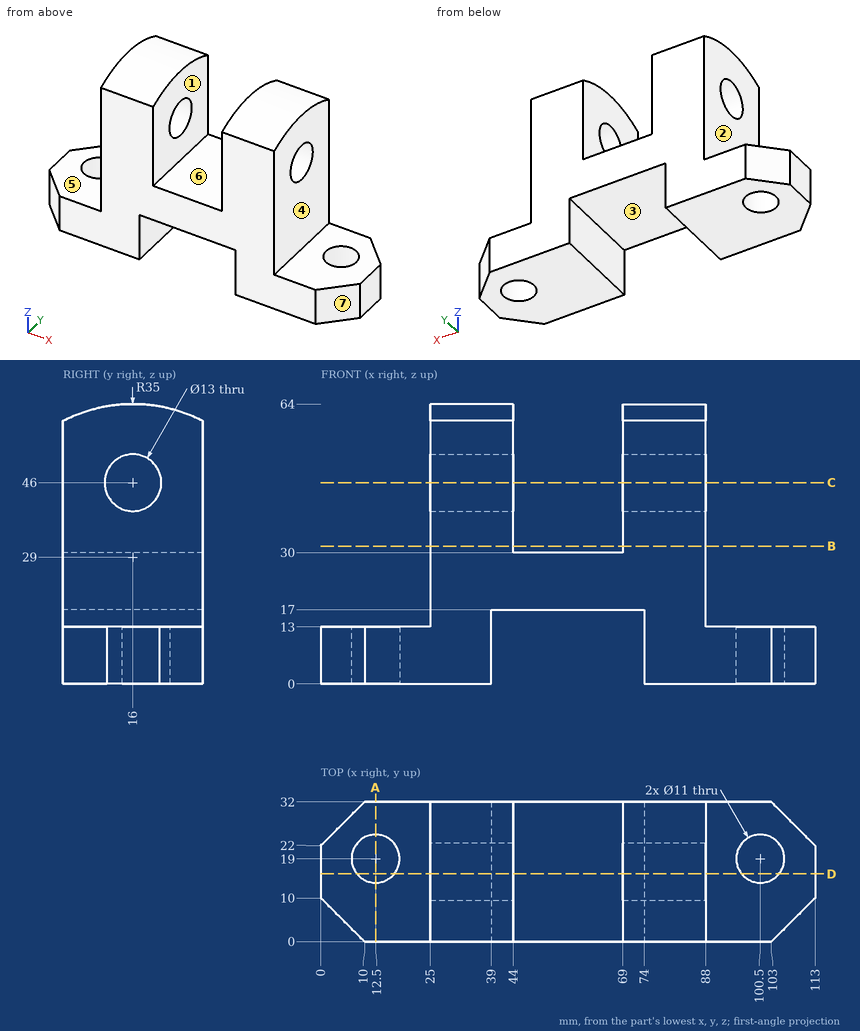
Drawing for the job (mm, zero at the part's lowest x, y, z). A direction names the side the tool comes from. Give positions to 0.01 mm unless a question says otherwise; leave off trailing zeros. Write each loop counter-clockwise with the first axis right and the second up, starting at its lowest first coordinate (ties: lowest second). Pieces come first, ordered by that corner, then holes. Notation, with made-up numbers: M 51.5,74.25 L 62.5,74.25 A25 ccw 62.5,111.25 Z; hole C -16.75,47 d1. An arc over 180 degrees is marked long. Return JSON: item names as keys, results as strings. Group by question number.
(1) Band-saw the part on B-B (z = 31.5). Give the cut face in (x, y).
(2) Band-saw the part on A-A (x = 12.5). Give the cut face in (y, z), and give its area (3 significant figures).
(3) Flat gauge pins, fed straight in: pin 1 Ø10 at (x, y) = (100.5, 19) entering from +Z; pin 2 Ø7.5 at (x, y) = (52, 16) entering from +Z; pin 3 Ø4 at (y, z) = (22, 17.5) entering from +X; pin 4 Ø9.5 at (x, y) = (48, 21.5) entering from -Z. Where does each tip first touch, or does it go through?
(4) 3-axis set-ups, long thin cutter, end or side, ignore diameter. For the marked faces 1, 2, 3 and 4: which of +Z, -Z, +X, -X, +Y, -Y reach the whole face in a straight line?
(5) Drill centre lines: L1, parallel to Y at x = 100.5, z = 4; L2, parallel to X at y = 10, z = 58.5; L3, parallel to X at y = 26, z = 13.5. Where is each one in solid material? Low to high. Write a range as [from, to].
(6) Mould opens along X. For the marked faces 5, 6 and 7 say: pulls with the +X half, pulls with the -X half, needs draft (parallel to the pull), parting line crosses it, or undercut.
(7) Band-saw the part on D-D (y = 15.5). State how many separate pieces and enclosed holes the cut face has, and give its area (3 significant figures).
(8) Band-saw the part on C-C (z = 46). Give the cut face in (x, y).
Entries:
{
 "1": {"outline": "M 25,0 L 44,0 L 44,32 L 25,32 Z; M 69,0 L 88,0 L 88,32 L 69,32 Z"},
 "2": {"outline": "M 0,0 L 13.5,0 L 13.5,13 L 0,13 Z; M 24.5,0 L 32,0 L 32,13 L 24.5,13 Z", "area": "273 mm^2"},
 "3": {"pin 1": "passes through", "pin 2": "stops at z = 30", "pin 3": "stops at x = 88", "pin 4": "stops at z = 17"},
 "4": {"face 1": "+Z, +Y, -Y", "face 2": "+Z, -X, +Y, -Y", "face 3": "-Z, +Y, -Y", "face 4": "+Z, +X, +Y, -Y"},
 "5": {"L1": "y = [0, 13.5], [24.5, 32]", "L2": "x = [25, 44], [69, 88]", "L3": "x = [25, 39], [74, 88]"},
 "6": {"face 5": "needs draft", "face 6": "undercut", "face 7": "pulls with the +X half"},
 "7": {"separate pieces": "5", "enclosed holes": "0", "area": "2,520 mm^2"},
 "8": {"outline": "M 25,0 L 44,0 L 44,9.5 L 25,9.5 Z; M 25,22.5 L 44,22.5 L 44,32 L 25,32 Z; M 69,0 L 88,0 L 88,9.5 L 69,9.5 Z; M 69,22.5 L 88,22.5 L 88,32 L 69,32 Z"}
}
